from build123d import *

# Parameters (mm, degrees)
SKETCH1_R           = 1.25
BOSS_EXTRUDE2_DEPTH = 1.6
SKETCH2_W           = 15
SKETCH2_H           = 15.35
BOSS_EXTRUDE3_DEPTH = 0.66
SKETCH3_W           = 5.3
SKETCH3_H           = 7.54
BOSS_EXTRUDE4_DEPTH = 2.5
FILLET1_R           = 0.5
FILLET2_R           = 1.5
SKETCH4_W           = 5.3
SKETCH4_H           = 7.54
BOSS_EXTRUDE5_DEPTH = 2.5
FILLET3_R           = 0.5
FILLET4_R           = 1.5
SKETCH5_W           = 7.22
SKETCH5_H           = 21.3
SKETCH5_W_2         = 23.6
SKETCH5_H_2         = 17.5
BOSS_EXTRUDE6_DEPTH = 3.45
FILLET5_R           = 1


with BuildPart() as part:
    # Sketch1 → Boss-Extrude2 (new body)
    with BuildSketch(Plane.XY):
        Polygon((0, 0), (53, 0), (53, 3.62), (91.22, 3.62), (91.22, 19.27), (53, 19.27), (53, 23), (0, 23), align=None)
        with Locations((40.6, 2.5)):
            Circle(SKETCH1_R, mode=Mode.SUBTRACT)
        with Locations((18.05, 2.5)):
            Circle(SKETCH1_R, mode=Mode.SUBTRACT)
    extrude(amount=BOSS_EXTRUDE2_DEPTH)

    # Sketch2 → Boss-Extrude3 (add)
    with BuildSketch(Plane(origin=(0, 0, 0), x_dir=(-1, 0, 0), z_dir=(0, 0, -1))):
        with Locations((-64.62, 11.445)):
            Rectangle(SKETCH2_W, SKETCH2_H)
    extrude(amount=BOSS_EXTRUDE3_DEPTH)

    # Sketch3 → Boss-Extrude4 (add)
    with BuildSketch(Plane.XY.offset(1.6)):
        with Locations((89.47, 11.89)):
            Rectangle(SKETCH3_W, SKETCH3_H)
    extrude(amount=BOSS_EXTRUDE4_DEPTH)

    # Fillet1
    fillet1_edges = [part.edges().sort_by_distance(p)[0] for p in [
        (89.47, 15.66, 4.1),
        (89.47, 8.12, 4.1),
    ]]
    fillet(fillet1_edges, radius=FILLET1_R)

    # Fillet2
    fillet2_edges = [part.edges().sort_by_distance(p)[0] for p in [
        (91.67, 15.66, 1.6),
        (91.67, 8.12, 1.6),
    ]]
    fillet(fillet2_edges, radius=FILLET2_R)

    # Sketch4 → Boss-Extrude5 (add)
    with BuildSketch(Plane(origin=(0, 0, 0), x_dir=(-1, 0, 0), z_dir=(0, 0, -1))):
        with Locations((-1.75, 11.47)):
            Rectangle(SKETCH4_W, SKETCH4_H)
    extrude(amount=BOSS_EXTRUDE5_DEPTH)

    # Fillet3
    fillet3_edges = [part.edges().sort_by_distance(p)[0] for p in [
        (1.75, 15.24, -2.5),
        (1.75, 7.7, -2.5),
    ]]
    fillet(fillet3_edges, radius=FILLET3_R)

    # Fillet4
    fillet4_edges = [part.edges().sort_by_distance(p)[0] for p in [
        (-0.45, 15.24, 0),
        (-0.45, 7.7, 0),
    ]]
    fillet(fillet4_edges, radius=FILLET4_R)

    # Sketch5 → Boss-Extrude6 (add)
    with BuildSketch(Plane.XY.offset(1.6)):
        with Locations((47.39, 11.35)):
            Rectangle(SKETCH5_W, SKETCH5_H)
        with Locations((65.1, 11.85)):
            Rectangle(SKETCH5_W_2, SKETCH5_H_2)
    extrude(amount=BOSS_EXTRUDE6_DEPTH)

    # Fillet5
    # the kernel refuses this fillet: 1 mm, written as the material it adds along each edge
    with BuildSketch(Plane(origin=(53, 19.27, 0), x_dir=(0, 1, 0), z_dir=(0, 0, 1)), Plane(origin=(53, 3.62, 0), x_dir=(1, 0, 0), z_dir=(0, 0, 1))) as fillet5_piece_1:
        with BuildLine():
            CenterArc((FILLET5_R, -FILLET5_R), FILLET5_R, 90, 90)
            Line((0, -FILLET5_R), (0, 0))
            Line((0, 0), (FILLET5_R, 0))
        make_face()
    extrude(amount=1.6)
    # the kernel refuses this fillet: 1 mm, written as the material it takes off along each edge
    with BuildSketch(Plane(origin=(0, 23, -2.5), x_dir=(1, 0, 0), z_dir=(0, 0, 1))) as fillet5_2_piece_1:
        with BuildLine():
            CenterArc((FILLET5_R, -FILLET5_R), FILLET5_R, 90, 90)
            Line((0, -FILLET5_R), (0, 0))
            Line((0, 0), (FILLET5_R, 0))
        make_face()
    extrude(amount=6.6, mode=Mode.SUBTRACT)
    with BuildSketch(Plane(origin=(53, 23, -2.5), x_dir=(-1, 0, 0), z_dir=(0, 0, 1)), Plane(origin=(91.22, 19.27, -2.5), x_dir=(-1, 0, 0), z_dir=(0, 0, 1)), Plane(origin=(91.22, 3.62, -2.5), x_dir=(0, 1, 0), z_dir=(0, 0, 1)), Plane(origin=(53, 0, -2.5), x_dir=(0, 1, 0), z_dir=(0, 0, 1)), Plane(origin=(0, 0, -2.5), x_dir=(1, 0, 0), z_dir=(0, 0, 1))) as fillet5_2_piece_2:
        with BuildLine():
            CenterArc((FILLET5_R, FILLET5_R), FILLET5_R, 180, 90)
            Line((0, FILLET5_R), (0, 0))
            Line((0, 0), (FILLET5_R, 0))
        make_face()
    extrude(amount=6.6, mode=Mode.SUBTRACT)


solid = part.part
Verification items for the finished model (mm, model axes). A direction names the side the tool comes from. Coordinates: 2 decimals unless noted, no trailing zeros. Loops run counter-clockwise (first coordinate to the right, second up) from the corner with the lowest first, then second, coordinate; pieces in that order, holes last. Notation, with made-up numbers: (7, 78.25) -> (11, 78.25) arc R20 cw to (11, 106.25) -> close; hole circle Ø5 at (66.5, 77). An arc over 180 degrees is marked (long way). Answer as CSV lines item,"result".
1) Thickness scan on L1, parallel to X at y = 10.75, z = 3.5; L2, parallel to Y at x = 18.05, z = 0.55; L3, parallel to X at y = 9.5, z = -0.5. Record the ranges inside material, lowest first. Write a range as from..to.
Found:
L1,"x = 43.78..51, 53.3..76.9, 86.82..92.12"
L2,"y = 0..1.25, 3.75..23"
L3,"x = -0.9..4.4, 57.12..72.12"
2) Tool access check on faces 1 (the flat face through (47, 0.7, 3)), 2 (the flat face through (72, 19.27, 1)), 3 (the flat face through (65, 12, -0.66)), 4 (the flat face through (89, 15.66, 3)), 5 (the flat face through (89, 8.12, 3)). Record the directions out of +Z, -Z, +X, -X, +Y, -Y that give a thin tool (end or side, any length) a straight path to the whole face; none if there is none.
Found:
face 1,"+Z, +X, -X, -Y"
face 2,"-Z, +X, +Y"
face 3,"-Z, +X, +Y, -Y"
face 4,"+Z, +X, +Y"
face 5,"+Z, +X, -Y"
3) Depth check by flat-ended pin: pin 1 (2 mm diameter, centred on x = 40.6, y = 2.5, fed in from -Z) (3 decimals); pin 2 (2 mm diameter, centred on x = 0.5, z = -1.5, fed in from -Y); pin 3 (1.5 mm diameter, centred on y = 16, z = 3.5, fed in from -X); pin 4 (4 mm diameter, centred on x = 63, z = 4, fed in from +Y). Enter the tip coordinate at first touch or a pass-through.
Found:
pin 1,"passes through"
pin 2,"stops at y = 7.7"
pin 3,"stops at x = 43.78"
pin 4,"stops at y = 20.6"
4) Cross-section at C-C, the plane x = 30. Record the cut outline in (y, z), then the cut area to 3 significant figures.
Found:
outline,"(0, 0) -> (23, 0) -> (23, 1.6) -> (0, 1.6) -> close"
area,"36.8 mm2"
5) Cross-section at B-B, the plane y = 10.5. Record the cut outline in (x, z).
Found:
outline,"(-0.9, -2.5) -> (4.4, -2.5) -> (4.4, 0) -> (57.12, 0) -> (57.12, -0.66) -> (72.12, -0.66) -> (72.12, 0) -> (91.22, 0) -> (91.22, 1.6) -> (92.12, 1.6) -> (92.12, 4.1) -> (86.82, 4.1) -> (86.82, 1.6) -> (76.9, 1.6) -> (76.9, 5.05) -> (53.3, 5.05) -> (53.3, 1.6) -> (51, 1.6) -> (51, 5.05) -> (43.78, 5.05) -> (43.78, 1.6) -> (0, 1.6) -> (0, 0) -> (-0.9, 0) -> close"
6) Cross-section at A-A, the plane x = 40.6. Record the cut outline in (y, z), then the cut area to 3 significant figures.
Found:
outline,"(0, 0) -> (1.25, 0) -> (1.25, 1.6) -> (0, 1.6) -> close; (3.75, 0) -> (23, 0) -> (23, 1.6) -> (3.75, 1.6) -> close"
area,"32.8 mm2"
7) Release check for a two-part mould opening along Y. For faces 6 (the flat face through (2, 7.7, -1)), 7 (the flat face through (-0.9, 11, -1)), 8 (the cylindrical face through (16.8, 2.55, 0.79)) record: +Y half, -Y half, draft (parallel to the pull), parting line (faces both ways), or undercut.
Found:
face 6,"-Y half"
face 7,"draft"
face 8,"undercut"
